Design review of the part shown in the three views and the two pictorial views. Dimensions are in mm from the part's minimum x, y and z. Give positions to 0.01 mm unless a question says otherwise; leave off trailing zeros. Loops run counter-clockwise (first coordinate to the right, second up) from the corner with the lowest first, then second, coordinate; pieces in that order, holes last. Notation, with made-up numbers: (34, -27.75) -> (47, -27.75) arc R25 ccw to (47, 7.25) -> close; hole circle Ø7 at (35, -28). An arc over 180 degrees is marked (long way). Use CSV: the item, a comma, the result in double quotes. Start each with the question number.
Item 1: The part is to be moulded in two halves that separate along Z. For the marked faces 1, 2 and 3, say which applies: +Z half, -Z half, draft (parallel to the pull), parting line (faces both ways), or undercut.
Item 2: We need section C-C (x = 10). State the section outline as (y, z) points (3 decimals).
Item 3: We need section A-A (z = 62.23). State the section outline as (x, y) points (3 decimals), plus the area to 3 significant figures.
Item 4: We need section B-B (y = 9.25). Count the separate pieces of the cut face and the enclosed holes in it, plus the area to 3 significant figures.
Item 5: Clearance check with flat-ended pins moving along their axes: pin 1 (4 mm diameter, centred on x = 35, y = 3.5, fed in from +Z); pin 2 (5 mm diameter, centred on y = 9, z = 78, fed in from -X); pin 3 (2 mm diameter, centred on x = 80, y = 11, fed in from +Z). State where each tip first meets the part, or that it passes through.
Item 6: Wall thickness on line 1 along Z through (x, y) = (49.5, 6.75); line 2 along X through (y, z) = (8.25, 31); line 3 along X through (y, z) = (9, 62): over which ranges is each line inside the solid? List them lowest first. Write a range as from..to.
Item 7: We need section D-D (z = 9). State the section outline as (x, y) points (3 decimals).
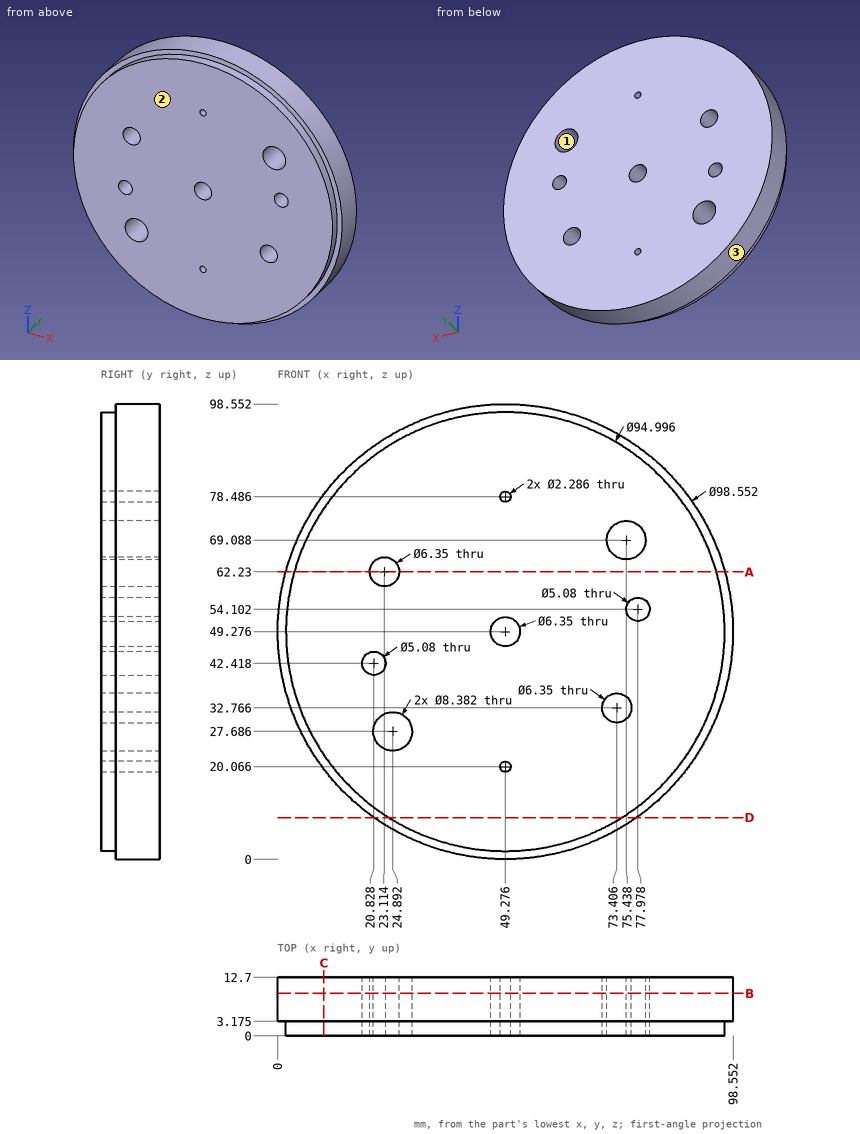
Results found:
1,face 1,"undercut"
1,face 2,"draft"
1,face 3,"parting line"
2,outline,"(0, 22.565) -> (3.175, 22.565) -> (3.175, 19.518) -> (12.7, 19.518) -> (12.7, 79.034) -> (3.175, 79.034) -> (3.175, 75.987) -> (0, 75.987) -> close"
3,outline,"(1.733, 3.175) -> (3.579, 3.175) -> (3.579, 0) -> (19.939, 0) -> (19.939, 12.7) -> (1.733, 12.7) -> close; (26.289, 0) -> (94.973, 0) -> (94.973, 3.175) -> (96.819, 3.175) -> (96.819, 12.7) -> (26.289, 12.7) -> close"
3,area,"1,120 mm²"
4,separate pieces,"1"
4,enclosed holes,"9"
4,area,"7,370 mm²"
5,pin 1,"z = 97"
5,pin 2,"x = 7.56"
5,pin 3,"z = 88.58"
6,line 1,"0..18.95, 21.19..46.11, 52.44..77.37, 79.61..98.55"
6,line 2,"3.51..22.33, 27.46..70.77, 76.04..95.04"
6,line 3,"1.67..19.95, 26.28..96.88"
7,outline,"(20.886, 3.175) -> (24.099, 3.175) -> (24.099, 0) -> (74.453, 0) -> (74.453, 3.175) -> (77.666, 3.175) -> (77.666, 12.7) -> (20.886, 12.7) -> close"
